Input: part model. Units: mm. Frame: model coordinates. A direction names the side the tool comes from. Round coordinates to 2 decimals unless told otherwise and drop trailing zeros. Order: outer loops, then holes, each group sorted by start corner. A loop starts at its lowest first (then second) coordinate and runs counter-clockwise, first axis right, second up. Notation, with made-up numbers: (12, 66) - (52, 66) arc R20 cw to (52, 87) - close; hole circle Ø4 at (2, 51.5). An arc over 180 degrees is marked (long way). One line per item, written item: value. Start each with the question number.
from build123d import *

# Parameters (mm, degrees)
SKETCH1_W           = 12.7
SKETCH1_H           = 12.7
BOSS_EXTRUDE1_DEPTH = 2.54
FILLET1_R           = 0.635
SHELL1_START        = 0.635
SHELL1_OUTLINE_W    = 1.905
SHELL1_OUTLINE_H    = 11.43
SHELL1_DEPTH        = 11.43
SKETCH2_R           = 2.54
BOSS_EXTRUDE2_DEPTH = 1.905
BOSS_EXTRUDE4_DEPTH = 0.00254


# Read off the part's stored shape, not the designer's step: Shell1
with BuildPart() as part:
    # Sketch1 → Boss-Extrude1 (new body)
    with BuildSketch(Plane(origin=(0, 0, 0), x_dir=(1, 0, 0), z_dir=(0, 1, 0))):
        with Locations((6.35, 6.35)):
            Rectangle(SKETCH1_W, SKETCH1_H)
    extrude(amount=BOSS_EXTRUDE1_DEPTH)

    # Fillet1
    fillet1_edges = [part.edges().sort_by_distance(p)[0] for p in [
        (0, 1.27, -12.7),
        (12.7, 1.27, -12.7),
        (12.7, 1.27, 0),
        (0, 1.27, 0),
    ]]
    fillet(fillet1_edges, radius=FILLET1_R)

    # Shell1 outline → Shell1 (cut)
    with BuildSketch(Plane.YZ.offset(SHELL1_START)):
        with Locations((0.9525, -6.35)):
            Rectangle(SHELL1_OUTLINE_W, SHELL1_OUTLINE_H)
    extrude(amount=SHELL1_DEPTH, mode=Mode.SUBTRACT)

    # Sketch2 → Boss-Extrude2 (add)
    with BuildSketch(Plane(origin=(0, 1.905, 0), x_dir=(-1, 0, 0), z_dir=(0, -1, 0))):
        with Locations(Location((-6.35, 6.35, 0), (0, 0, 270))):
            Circle(SKETCH2_R)
    extrude(amount=BOSS_EXTRUDE2_DEPTH)

    # Sketch4 → Boss-Extrude4 (add)
    # profile 1 of 2: a face of its own
    with BuildSketch(Plane(origin=(0, 2.54, 0), x_dir=(1, 0, 0), z_dir=(0, 1, 0))):
        Polygon((6.480510817, 5.974210256), (7.074551282, 5.974210256), (7.074551282, 3.898248718), (7.359487179, 3.898248718), (7.359487179, 3.369082051), (7.074551282, 3.369082051), (7.074551282, 2.7178), (6.504679487, 2.7178), (6.504679487, 3.369082051), (5.161410256, 3.369082051), (5.161410256, 3.94595004), align=None)
        Polygon((6.504679487, 3.898248718), (6.504679487, 4.978842668), (5.801880008, 3.898248718), align=None, mode=Mode.SUBTRACT)
    # profile 2 of 2: a face of its own
    with BuildSketch(Plane(origin=(0, 2.54, 0), x_dir=(1, 0, 0), z_dir=(0, 1, 0))):
        with BuildLine():
            Line((7.406984976, 10.335998798), (6.991665465, 9.935307692))
            add(Edge.make_bspline(
                [(6.991665465, 9.935307692), (6.968220024, 9.957896469), (6.922854486, 10.001604413), (6.851968783, 10.059827369), (6.781357064, 10.108976166), (6.711092446, 10.149588351), (6.640799627, 10.181124743), (6.570421611, 10.203546558), (6.500157891, 10.217583932), (6.453231922, 10.219364448), (6.430061899, 10.22024359)],
                knots=[0, 0, 0, 0, 1.208861562, 2.33907556, 3.402820298, 4.400980881, 5.349191832, 6.258141005, 7.139945025, 8, 8, 8, 8], degree=3))
            add(Edge.make_bspline(
                [(6.430061899, 10.22024359), (6.403899471, 10.219170975), (6.353552661, 10.217106842), (6.281800477, 10.200625662), (6.218083395, 10.171963441), (6.162978001, 10.1335672), (6.118660061, 10.08737089), (6.085670238, 10.036873816), (6.065418702, 9.982146492), (6.063012994, 9.944162193), (6.061807692, 9.92513141)],
                knots=[0, 0, 0, 0, 1.198011544, 2.305445805, 3.348962256, 4.381113563, 5.363569282, 6.263566672, 7.130017225, 8, 8, 8, 8], degree=3))
            add(Edge.make_bspline(
                [(6.061807692, 9.92513141), (6.062942346, 9.908653977), (6.065271259, 9.874833543), (6.08412075, 9.82517461), (6.11232136, 9.775299071), (6.138383978, 9.745137076), (6.152122196, 9.729237981)],
                knots=[0, 0, 0, 0, 0.894516561, 1.836022459, 2.859316659, 4, 4, 4, 4], degree=3))
            add(Edge.make_bspline(
                [(6.152122196, 9.729237981), (6.160244287, 9.720816207), (6.177567552, 9.702853763), (6.208320254, 9.677594331), (6.244828496, 9.652473945), (6.286427709, 9.626009569), (6.334076496, 9.599858268), (6.386982478, 9.572031842), (6.4461068, 9.54521439), (6.487487603, 9.527340869), (6.508928085, 9.518080128)],
                knots=[0, 0, 0, 0, 0.672423156, 1.434182798, 2.28314655, 3.220082228, 4.268069212, 5.407712864, 6.656867891, 8, 8, 8, 8], degree=3))
            add(Edge.make_bspline(
                [(6.508928085, 9.518080128), (6.547123945, 9.501624615), (6.620529049, 9.470000279), (6.725949021, 9.423048644), (6.821745388, 9.377334714), (6.908362629, 9.333599875), (6.985371716, 9.291637921), (7.053234273, 9.251918102), (7.110960799, 9.212858211), (7.176358415, 9.165369813), (7.245332068, 9.101127918), (7.319697388, 9.019919388), (7.382052409, 8.929969443), (7.434496037, 8.833656469), (7.475970735, 8.730809102), (7.506000976, 8.621840061), (7.524224787, 8.506579255), (7.526188983, 8.42758935), (7.527192308, 8.387240785)],
                knots=[0, 0, 0, 0, 1.218452834, 2.341632252, 3.380669879, 4.327878116, 5.183951769, 5.949833714, 6.63028248, 7.225317665, 8.315786147, 9.384546881, 10.445973047, 11.51321668, 12.591625589, 13.68712373, 14.81856753, 16, 16, 16, 16], degree=3))
            add(Edge.make_bspline(
                [(7.527192308, 8.387240785), (7.525940527, 8.346682546), (7.523476092, 8.266833747), (7.504812176, 8.149311253), (7.472571433, 8.036846212), (7.429153295, 7.929917836), (7.374984908, 7.831254365), (7.31426383, 7.741649541), (7.245676289, 7.662999272), (7.181542739, 7.60682825), (7.126266053, 7.566022086), (7.079408572, 7.539362519), (7.029180829, 7.512893987), (6.974279808, 7.488884305), (6.915217227, 7.466725999), (6.851680833, 7.446436031), (6.784149797, 7.427141632), (6.737109705, 7.416846646), (6.713089744, 7.411589744)],
                knots=[0, 0, 0, 0, 1.398055402, 2.752413464, 4.089819795, 5.424146338, 6.722736095, 7.963569404, 9.149738937, 10.309787565, 10.896110825, 11.515406893, 12.166006826, 12.853269453, 13.579614796, 14.340134636, 15.152427224, 16, 16, 16, 16], degree=3))
            Line((6.713089744, 7.411589744), (6.713089744, 6.841717949))
            Line((6.713089744, 6.841717949), (6.306038462, 6.841717949))
            Line((6.306038462, 6.841717949), (6.306038462, 7.411589744))
            add(Edge.make_bspline(
                [(6.306038462, 7.411589744), (6.260932407, 7.417508865), (6.173627208, 7.428965643), (6.048973026, 7.459844727), (5.933431761, 7.497036363), (5.863209037, 7.532393856), (5.82902524, 7.549605569)],
                knots=[0, 0, 0, 0, 1.092056374, 2.113733945, 3.081782489, 4, 4, 4, 4], degree=3))
            add(Edge.make_bspline(
                [(5.82902524, 7.549605569), (5.784421922, 7.575319651), (5.694521215, 7.627147952), (5.567652028, 7.720202965), (5.443690251, 7.822749518), (5.367680431, 7.900192292), (5.329115385, 7.939484375)],
                knots=[0, 0, 0, 0, 0.970088211, 1.955271939, 2.962567826, 4, 4, 4, 4], degree=3))
            Line((5.329115385, 7.939484375), (5.73807472, 8.347807692))
            add(Edge.make_bspline(
                [(5.73807472, 8.347807692), (5.770276914, 8.315531916), (5.832553047, 8.253113482), (5.930208341, 8.170258717), (6.026937688, 8.099683859), (6.123133593, 8.042123916), (6.21841229, 7.996807875), (6.313137257, 7.964752249), (6.40716107, 7.944584507), (6.469824943, 7.942018876), (6.500659856, 7.94075641)],
                knots=[0, 0, 0, 0, 1.232518957, 2.38358023, 3.459285847, 4.467107529, 5.410929513, 6.306558082, 7.166710731, 8, 8, 8, 8], degree=3))
            add(Edge.make_bspline(
                [(6.500659856, 7.94075641), (6.530935033, 7.942287354), (6.590433781, 7.945296064), (6.676251693, 7.970961733), (6.754438188, 8.014226678), (6.824451013, 8.071818039), (6.882924302, 8.140474874), (6.926114925, 8.217254316), (6.952937787, 8.300259042), (6.955847074, 8.357998183), (6.957320513, 8.387240785)],
                knots=[0, 0, 0, 0, 1.025332292, 2.015049702, 3.006124463, 4.038216902, 5.073984904, 6.04617681, 7.010465453, 8, 8, 8, 8], degree=3))
            add(Edge.make_bspline(
                [(6.957320513, 8.387240785), (6.95646201, 8.411933563), (6.954785019, 8.460168152), (6.938095616, 8.529934505), (6.911632454, 8.595452748), (6.88533712, 8.634212047), (6.872094151, 8.653732171)],
                knots=[0, 0, 0, 0, 1.039339221, 2.030233321, 3.007977686, 4, 4, 4, 4], degree=3))
            add(Edge.make_bspline(
                [(6.872094151, 8.653732171), (6.85460202, 8.673362669), (6.816189839, 8.716470638), (6.740466296, 8.774265663), (6.645219094, 8.832335499), (6.573483267, 8.868013356), (6.535004808, 8.887150641)],
                knots=[0, 0, 0, 0, 0.762317005, 1.674024744, 2.752367564, 4, 4, 4, 4], degree=3))
            add(Edge.make_bspline(
                [(6.535004808, 8.887150641), (6.494507252, 8.906433078), (6.416597652, 8.943528822), (6.304602291, 8.997049085), (6.203256868, 9.048626278), (6.112557984, 9.097686427), (6.03159058, 9.142731993), (5.960729388, 9.184249859), (5.900795306, 9.224016823), (5.83450108, 9.27124253), (5.764387026, 9.331778858), (5.691098847, 9.407825341), (5.628662473, 9.487993783), (5.578981708, 9.573423124), (5.539805424, 9.661899474), (5.512543165, 9.753617062), (5.495251156, 9.847946671), (5.493048251, 9.91191248), (5.491935897, 9.944211939)],
                knots=[0, 0, 0, 0, 1.361149963, 2.618593809, 3.766618961, 4.811512794, 5.747589985, 6.578416214, 7.302870291, 7.929605856, 9.047509489, 10.107720061, 11.130736737, 12.122694611, 13.099282469, 14.059974503, 15.020386449, 16, 16, 16, 16], degree=3))
            add(Edge.make_bspline(
                [(5.491935897, 9.944211939), (5.492688489, 9.970752491), (5.494175897, 10.023206783), (5.505434517, 10.100481592), (5.522750824, 10.175049255), (5.548766759, 10.246263408), (5.581362042, 10.314610672), (5.620802687, 10.380506472), (5.6682686, 10.442870868), (5.722186861, 10.501770993), (5.78128424, 10.555933143), (5.844845686, 10.604219102), (5.912333412, 10.645653847), (5.983778264, 10.680011213), (6.058992906, 10.707624067), (6.137825565, 10.728257196), (6.220507462, 10.743532862), (6.277140501, 10.747424489), (6.306038462, 10.749410256)],
                knots=[0, 0, 0, 0, 1.004170626, 1.984625641, 2.949958411, 3.896703334, 4.847824684, 5.812490235, 6.7978582, 7.808834457, 8.831147227, 9.827755371, 10.825493475, 11.823199312, 12.823418834, 13.853042784, 14.904478961, 16, 16, 16, 16], degree=3))
            Line((6.306038462, 10.749410256), (6.306038462, 10.952935897))
            Line((6.306038462, 10.952935897), (6.713089744, 10.952935897))
            Line((6.713089744, 10.952935897), (6.713089744, 10.749410256))
            add(Edge.make_bspline(
                [(6.713089744, 10.749410256), (6.746474507, 10.740874198), (6.811234543, 10.724315883), (6.903809354, 10.69417972), (6.987944372, 10.65820288), (7.067293727, 10.617748164), (7.145681965, 10.56733025), (7.227556159, 10.503669804), (7.31605682, 10.425644759), (7.375483722, 10.367055847), (7.406984976, 10.335998798)],
                knots=[0, 0, 0, 0, 1.007023709, 1.953432773, 2.841901989, 3.678835315, 4.553739984, 5.561316369, 6.707292646, 8, 8, 8, 8], degree=3))
        make_face()
    extrude(amount=BOSS_EXTRUDE4_DEPTH)


solid = part.part
Item 1: Reachability of faces 1 (the face through (7, 2.543, -9)), 2 (the face through (6, 1, -0.635)) from +Z, -Z, +X, -X, +Y, -Y: full face, straight path, thin tool, end or side. Return the list, or none.
Item 2: Section query D-D on z = -2.5. Return loops of the section in (x, y) (3 decimals), and give its area (3 significant figures).
Item 3: Section query A-A on y = 1. Return loops of the section in (x, z) (3 decimals).
Item 4: Pull-direction query (X, two-part tool) for faces 3 (the face through (12.7, 1, -6)), 4 (the face through (6, 1, -12.065)), 5 (the face through (6, 2.54, -6)), 6 (the face through (0.635, 1, -6)); classes: released by +X, released by -X, zero draft, split by the parting line, or undercut.
Item 5: Section query C-C on x = 2.75. Return loops of the section in (y, z) (3 decimals), and give its area (3 significant figures).
Item 6: Line query: L1, parallel to X at y = 1.2, z = -6.25 (3 decimals); L2, parallel to X at y = 1.3, z = -9 (3 decimals); L3, parallel to X at y = 1, z = -4.75 (3 decimals). Output: solid intervals per line, ascending.
Item 7: Section query B-B on z = -6.35. Return loops of the section in (x, y) (3 decimals).
Geometry results:
1. face 1: +Z, -Z, +X, -X, +Y
1. face 2: -Y
2. outline: (0, 0) - (0.635, 0) - (0.635, 1.905) - (12.065, 1.905) - (12.065, 0) - (12.7, 0) - (12.7, 2.54) - (0, 2.54) - close
2. area: 10.5 mm^2
3. outline: (0, -12.065) arc R0.635 ccw to (0.635, -12.7) - (12.065, -12.7) arc R0.635 ccw to (12.7, -12.065) - (12.7, -0.635) arc R0.635 ccw to (12.065, 0) - (0.635, 0) arc R0.635 ccw to (0, -0.635) - close; circle Ø5.08 at (6.35, -6.35); hole (0.635, -12.065) - (12.065, -12.065) - (12.065, -0.635) - (0.635, -0.635) - close
4. face 3: released by +X
4. face 4: undercut
4. face 5: zero draft
4. face 6: undercut
5. outline: (0, -12.7) - (2.54, -12.7) - (2.54, 0) - (0, 0) - (0, -0.635) - (1.905, -0.635) - (1.905, -12.065) - (0, -12.065) - close
5. area: 10.5 mm^2
6. L1: x = 0 to 0.635, 3.812 to 8.888, 12.065 to 12.7
6. L2: x = 0 to 0.635, 12.065 to 12.7
6. L3: x = 0 to 0.635, 4.377 to 8.323, 12.065 to 12.7
7. outline: (0, 0) - (0.635, 0) - (0.635, 1.905) - (3.81, 1.905) - (3.81, 0) - (8.89, 0) - (8.89, 1.905) - (12.065, 1.905) - (12.065, 0) - (12.7, 0) - (12.7, 2.54) - (0, 2.54) - close
